Input: part model. Units: mm. Frame: model coordinates. Face numbers are marked on the shaded views. A direction names the side the tool comes from. Coordinates: 2 decimals unless noted, no trailing zeros. Loops run counter-clockwise (first coordinate to the right, second up) from the corner with the lowest first, then second, coordinate; pieces in that order, holes last.
```python
from build123d import *

# Parameters (mm, degrees)
SM_BASE_FLANGE_1_DEPTH             = 16
SKETCH_3_R                         = 2.75
CUT_EXTRUDE_1_DEPTH                = 73.801098893
SKETCH_4_W                         = 12
SKETCH_4_H                         = 3.5
CUT_EXTRUDE_2_DEPTH                = 75.726166769
SM_EDGE_FLANGE_1_STRIP_W           = 9.4732
SM_EDGE_FLANGE_1_STRIP_H           = 2
SM_EDGE_FLANGE_1_STRIP_CUT_DEPTH   = 69.2634
SM_EDGE_FLANGE_1_STRIP_2_W         = 9.4732
SM_EDGE_FLANGE_1_STRIP_2_H         = 2
SM_EDGE_FLANGE_1_STRIP_CUT_2_DEPTH = 69.2634
SM_EDGE_FLANGE_1_DEPTH             = 69.2634
SM_EDGE_FLANGE_1_BEND_DEPTH        = 69.2634
M4X0_7_1_D                         = 3.3
M4X0_7_1_DEPTH                     = 10.1
M4X0_7_1_TIP                       = 0.991420021
CHAMFER_1_SIZE                     = 2


# Sheet-metal steps are written as plain solids
with BuildPart() as part:
    # Sketch 1 → 基体-法兰1 (new, symmetric)
    with BuildSketch(Plane.XY):
        with BuildLine():
            Line((0, 70), (0, 0.7366))
            ThreePointArc((0, 0.7366), (-0.215745145, 0.215745145), (-0.7366, 0))
            Line((-0.7366, 0), (-12, 0))
            Line((-12, 0), (-12, -2))
            Line((-12, -2), (-0.7366, -2))
            ThreePointArc((-0.7366, -2), (1.198468417, -1.198468417), (2, 0.7366))
            Line((2, 0.7366), (2, 70))
            Line((2, 70), (0, 70))
        make_face()
    extrude(amount=SM_BASE_FLANGE_1_DEPTH, both=True)

    # 草图3 → 切除-拉伸1 (cut, through all)
    with BuildSketch(Plane(origin=(0, 0, 0), x_dir=(1, 0, 0), z_dir=(0, 1, 0))):
        with Locations(Location((-7, 7, 0), (0, 0, 270))):
            Circle(SKETCH_3_R)
        with Locations(Location((-7, -7, 0), (0, 0, 270))):
            Circle(SKETCH_3_R)
    extrude(amount=-CUT_EXTRUDE_1_DEPTH, mode=Mode.SUBTRACT)

    # 草图4 → 切除-拉伸2 (cut, through all)
    with BuildSketch(Plane(origin=(0, 70, 0), x_dir=(1, 0, 0), z_dir=(0, 1, 0))):
        with Locations((-6, 14.25)):
            Rectangle(SKETCH_4_W, SKETCH_4_H)
        with Locations((-6, -14.25)):
            Rectangle(SKETCH_4_W, SKETCH_4_H)
    extrude(amount=-CUT_EXTRUDE_2_DEPTH, mode=Mode.SUBTRACT)

    # 边线-法兰1 strip (across the edge) → 边线-法兰1 strip cut (cut)
    with BuildSketch(Plane(origin=(2, 70, 16), x_dir=(0, 0, -1), z_dir=(0, -1, 0))):
        with Locations((-4, -1)):
            Rectangle(SM_EDGE_FLANGE_1_STRIP_W, SM_EDGE_FLANGE_1_STRIP_H)
    extrude(amount=SM_EDGE_FLANGE_1_STRIP_CUT_DEPTH, mode=Mode.SUBTRACT)

    # 边线-法兰1 strip 2 (across the edge) → 边线-法兰1 strip cut 2 (cut)
    with BuildSketch(Plane(origin=(2, 0.7366, -16), x_dir=(0, 0, 1), z_dir=(0, 1, 0))):
        with Locations((-4, -1)):
            Rectangle(SM_EDGE_FLANGE_1_STRIP_2_W, SM_EDGE_FLANGE_1_STRIP_2_H)
    extrude(amount=SM_EDGE_FLANGE_1_STRIP_CUT_2_DEPTH, mode=Mode.SUBTRACT)

    # 边线-法兰1 section (across the edge) → 边线-法兰1 (add)
    with BuildSketch(Plane(origin=(2, 70, 16), x_dir=(0, 0, -1), z_dir=(0, -1, 0))):
        with BuildLine():
            Line((-2, 0.7366), (-2, 10))
            Line((-2, 10), (0, 10))
            Line((0, 10), (0, 0.7366))
            ThreePointArc((0, 0.7366), (0.215745145, 0.215745145), (0.7366, 0))
            Line((0.7366, 0), (0.7366, -2))
            ThreePointArc((0.7366, -2), (-1.198468417, -1.198468417), (-2, 0.7366))
        make_face()
    extrude(amount=SM_EDGE_FLANGE_1_DEPTH)

    # 边线-法兰1 section 2 (across the edge) → 边线-法兰1 bend (add)
    with BuildSketch(Plane(origin=(2, 0.7366, -16), x_dir=(0, 0, 1), z_dir=(0, 1, 0))):
        with BuildLine():
            Line((-2, 0.7366), (-2, 10))
            Line((-2, 10), (0, 10))
            Line((0, 10), (0, 0.7366))
            ThreePointArc((0, 0.7366), (0.215745145, 0.215745145), (0.7366, 0))
            Line((0.7366, 0), (0.7366, -2))
            ThreePointArc((0.7366, -2), (-1.198468417, -1.198468417), (-2, 0.7366))
        make_face()
    extrude(amount=SM_EDGE_FLANGE_1_BEND_DEPTH)

    # M4x0.7 螺纹孔1
    with Locations(Plane(origin=(2, 0, 0), x_dir=(0, 0, -1), z_dir=(1, 0, 0))):
        with Locations((-5, 15), (5, 15)):
            Hole(M4X0_7_1_D / 2, depth=M4X0_7_1_DEPTH)
            with Locations((0, 0, -(M4X0_7_1_DEPTH + M4X0_7_1_TIP / 2))):  # 118° drill point
                Cone(0, M4X0_7_1_D / 2, M4X0_7_1_TIP, mode=Mode.SUBTRACT)

    # 倒角1
    chamfer_1_edges = [part.edges().sort_by_distance(p)[0] for p in [
        (12, 70, 17),
        (12, 0.7366, 17),
        (12, 0.7366, -17),
        (12, 70, -17),
        (-12, -1, -12.5),
        (-12, -1, 12.5),
    ]]
    chamfer(chamfer_1_edges, length=CHAMFER_1_SIZE)


solid = part.part
```
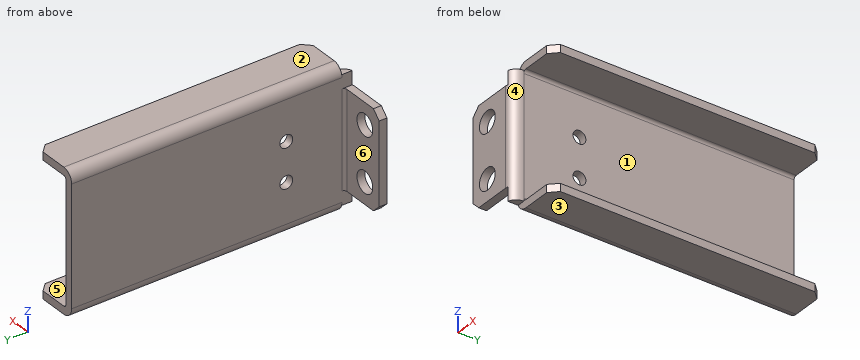
Item 1: Contact query for flat-ended pins moving along their axis: P1, Ø12, axis at x = 0, y = 56, coming from the -Z side; P2, Ø1.4, axis at x = 5, z = -16, coming from the -Y side; P3, Ø6, axis at x = -9.5, z = 10, coming from the +Y side; P4, Ø1.4, axis at x = -6, y = -0.5, coming from the -Z side. Output: stop coordinate, or through.
Result:
P1: stops at z = -18
P2: stops at y = 0.74
P3: stops at y = 0
P4: stops at z = -12.5
Item 2: Mould query, pull axis Z, two halves, no side actions, for the marked faces 1, 2 and 3. Classes: +Z half, -Z half, draft (parallel to the pull), parting line (faces both ways), or undercut.
Result:
face 1: undercut
face 2: +Z half
face 3: -Z half
Item 3: Line query: L1, parallel to Z at x = 9, y = 24; L2, parallel to X at y = 66, z = 0.5; L3, parallel to Y at x = -3.5, z = 4. Output: solid intervals per line, ascending.
Result:
L1: z = -18 to -16, 16 to 18
L2: x = 0 to 2
L3: y = -2 to 0
Item 4: Section query A-A (x = 7). Output: boundary loops of the cut face in (y, z).
Result:
outline: (0.74, -18) - (70, -18) - (70, -16) - (0.74, -16) - close; (0.74, 16) - (70, 16) - (70, 18) - (0.74, 18) - close
Item 5: Reachability of the marked faces 4, 5 and 6 from +Z, -Z, +X, -X, +Y, -Y: full face, straight path, thin tool, end or side. Return the list, or none.
Result:
face 4: +Z, -Z, +X, -Y
face 5: +X, +Y, -Y
face 6: +Z, -Z, -X, +Y
Item 6: Section query B-B (x = -7). Output: boundary loops of the cut face in (y, z).
Result:
outline: (-2, -12.5) - (0, -12.5) - (0, -9.75) - (-2, -9.75) - close; (-2, -4.25) - (0, -4.25) - (0, 4.25) - (-2, 4.25) - close; (-2, 9.75) - (0, 9.75) - (0, 12.5) - (-2, 12.5) - close
Item 7: Section query C-C (y = 15). Output: boundary loops of the cut face in (x, z).
Result:
outline: (0, -15.26) arc R2.74 ccw to (2.74, -18) - (12, -18) - (12, -16) - (2.74, -16) arc R0.74 cw to (2, -15.26) - (2, -6.65) - (0, -6.65) - close; (0, -3.35) - (2, -3.35) - (2, 3.35) - (0, 3.35) - close; (0, 6.65) - (2, 6.65) - (2, 15.26) arc R0.74 cw to (2.74, 16) - (12, 16) - (12, 18) - (2.74, 18) arc R2.74 ccw to (0, 15.26) - close
Item 8: Section query D-D (z = 5). Output: boundary loops of the cut face in (x, y).
Result:
outline: (-12, -2) - (-8.89, -2) - (-8.89, 0) - (-12, 0) - close; (-5.11, -2) - (-0.74, -2) arc R2.74 ccw to (2, 0.74) - (2, 13.35) - (0, 13.35) - (0, 0.74) arc R0.74 cw to (-0.74, 0) - (-5.11, 0) - close; (0, 16.65) - (2, 16.65) - (2, 70) - (0, 70) - close
